from build123d import *

# Parameters (mm, degrees)
SKETCH1_W           = 19
SKETCH1_H           = 6
BOSS_EXTRUDE1_DEPTH = 15
SKETCH2_W           = 23
SKETCH2_H           = 10
BOSS_EXTRUDE2_DEPTH = 2
SKETCH3_W           = 17
SKETCH3_H           = 4
BOSS_EXTRUDE3_DEPTH = 4
CUT_EXTRUDE1_DEPTH  = 4
FILLET1_R           = 1


with BuildPart() as part:
    # Sketch1 → Boss-Extrude1 (new body)
    with BuildSketch(Plane(origin=(0, 0, 0), x_dir=(1, 0, 0), z_dir=(0, 1, 0))):
        with Locations((-9.5, 3)):
            Rectangle(SKETCH1_W, SKETCH1_H)
    extrude(amount=BOSS_EXTRUDE1_DEPTH)

    # Sketch2 → Boss-Extrude2 (add)
    with BuildSketch(Plane(origin=(0, 15, 0), x_dir=(1, 0, 0), z_dir=(0, 1, 0))):
        with Locations((-9.5, 3)):
            Rectangle(SKETCH2_W, SKETCH2_H)
    extrude(amount=BOSS_EXTRUDE2_DEPTH)

    # Sketch3 → Boss-Extrude3 (add)
    with BuildSketch(Plane(origin=(0, 17, 0), x_dir=(1, 0, 0), z_dir=(0, 1, 0))):
        with Locations((-9.5, 3)):
            Rectangle(SKETCH3_W, SKETCH3_H)
    extrude(amount=BOSS_EXTRUDE3_DEPTH)

    # Sketch4 → Cut-Extrude1 (cut)
    with BuildSketch(Plane(origin=(0, 0, -5), x_dir=(-1, 0, 0), z_dir=(0, 0, -1))):
        with BuildLine():
            Line((1, 21), (1, 17))
            ThreePointArc((1, 17), (1.525373828, 19.234142662), (2.991374837, 21))
            Line((2.991374837, 21), (1, 21))
        make_face()
        with BuildLine():
            ThreePointArc((2.991374837, 21), (10.232075784, 18.010887947), (18, 17))
            Line((18, 17), (18, 21))
            Line((18, 21), (2.991374837, 21))
        make_face()
    extrude(amount=-CUT_EXTRUDE1_DEPTH, mode=Mode.SUBTRACT)

    # Fillet1
    fillet1_edges = [part.edges().sort_by_distance(p)[0] for p in [
        (-21, 17, -3),
        (-9.5, 17, 2),
        (2, 17, -3),
        (-9.5, 17, -8),
    ]]
    fillet(fillet1_edges, radius=FILLET1_R)


solid = part.part
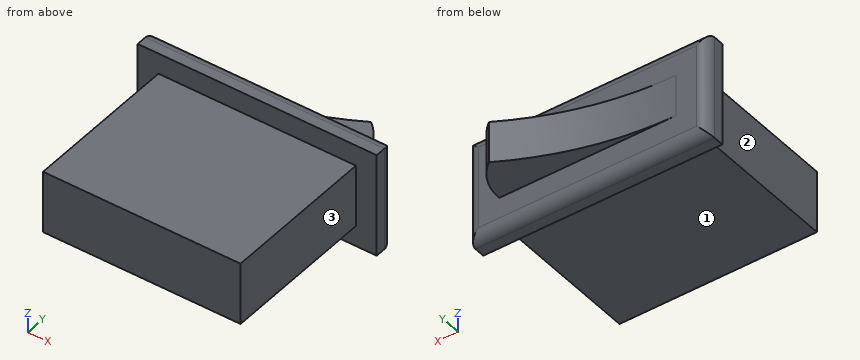
Build history of the part. All positions in model axes, mm. Face numbers are marked on the shaded views. A direction names the side the tool comes from. Give positions to 0.01 mm unless a question says otherwise; leave off trailing zeros. Write each loop counter-clockwise with the first axis right and the second up, starting at its lowest first coordinate (ties: lowest second). Pieces come first, ordered by that corner, then holes. Notation, with made-up numbers: (-15, 78) - (-5, 78) arc R20 cw to (-5, 102) - close; hole circle Ø2 at (32.25, 76). An arc over 180 degrees is marked (long way). Use one line per item in the form item = value. Start each with the question number.
1. Probe line 1 (X direction, y = 4, z = -4.75); line 2 (Y direction, x = -17.25, z = -0.75); line 3 (Y direction, x = -14, z = -7). List the from-to ranges inside material, lowest first. Write a range as [from, to].
2. Band-saw the part on C-C on x = -7.5. Write the cut outline in (y, z), plus the area to 3 significant figures.
3. Band-saw the part on B-B on y = 4.5. Write the cut outline in (x, z).
4. 3-axis set-ups, long thin cutter, end or side, ignore diameter. For the marked faces 1, 2 and 3: which of +Z, -Z, +X, -X, +Y, -Y reach the whole face in a straight line?
5. Drop flat-ended pins along their axis: pin 1 Ø2 at (x, y) = (-1, 11.5) entering from -Z; pin 2 Ø5 at (y, z) = (9, -3.5) entering from +X; pin 3 Ø1.5 at (x, y) = (-2.5, 17.5) entering from -Z. Give the stop position or say it passes through.
6. Band-saw the part on D-D on y = 17.5. Write the cut outline in (x, z) (3 decimals).
Conclusion:
q1.line_1 = [-19, 0]
q1.line_2 = [0, 17]
q1.line_3 = [15, 17]
q2.outline = (0, -6) - (15, -6) - (15, -8) - (16, -8) arc R1 ccw to (17, -7) - (17, -5) - (18.88, -5) - (18.88, -1) - (17, -1) - (17, 1) arc R1 ccw to (16, 2) - (15, 2) - (15, 0) - (0, 0) - close
q2.area = 117 mm²
q3.outline = (-19, -6) - (0, -6) - (0, 0) - (-19, 0) - close
q4.face_1 = -Z, +X, -X, -Y
q4.face_2 = +Z, -Z, -X, -Y
q4.face_3 = +Z, -Z, +X, -Y
q5.pin_1 = -6
q5.pin_2 = 0
q5.pin_3 = -7.66
q6.outline = (-12.499, -5) - (-1.025, -5) - (-1.025, -1) - (-12.499, -1) - close
